from build123d import *

# Parameters (mm, degrees)
CUT_EXTRUDE_1_DEPTH      = 135.169668703
CUT_EXTRUDE_1_DEPTH_BACK = 135.169668703
SKETCH_4_R               = 3
SKETCH_5_R               = 1.5
CUT_EXTRUDE_2_DEPTH      = 10
CHAMFER_1_SIZE           = 1


with BuildPart() as part:
    # 草图1 → 旋转1 (revolve)
    with BuildSketch(Plane.XY, mode=Mode.PRIVATE) as revolve_1_sk:
        Polygon((0, 0), (0, 8), (-73.934886909, 8), (-73.934886909, 7.5), (-75.934886909, 7.5), (-75.934886909, 12.5), (-84.5, 12.5), (-84.5, 8.5), (-86.5, 8.5), (-86.5, 9), (-118, 9), (-118, 7), (-120.5, 7), (-120.5, 8), (-133, 8), (-133, 0), align=None)
    revolve(revolve_1_sk.sketch.rotate(Axis((0, 0, 0), (1, 0, 0)), 90), axis=Axis((0, 0, 0), (1, 0, 0)))

    # 草图3 → 切除-旋转3 (revolve, cut)
    with BuildSketch(Plane.XY, mode=Mode.PRIVATE) as cut_revolve_3_sk:
        with BuildLine():
            Line((-133, 3.866025404), (-131.5, 3))
            Line((-131.5, 3), (-125, 3))
            Line((-125, 3), (-125, 1.5))
            Line((-125, 1.5), (-75, 1.5))
            ThreePointArc((-75, 1.5), (-73.939339828, 1.060660172), (-73.5, 0))
            Line((-73.5, 0), (-133, 0))
            Line((-133, 0), (-133, 3.866025404))
        make_face()
    revolve(cut_revolve_3_sk.sketch.rotate(Axis((-133, 0, 0), (1, 0, 0)), 90), axis=Axis((-133, 0, 0), (1, 0, 0)), mode=Mode.SUBTRACT)

    # 草图4 → 切除-拉伸1 (cut, two sides: drawn at the far end of the back side and taken through both)
    with BuildSketch(Plane.XY.offset(-CUT_EXTRUDE_1_DEPTH_BACK)):
        with Locations((-11.434886909, 0)):
            Circle(SKETCH_4_R)
    extrude(amount=CUT_EXTRUDE_1_DEPTH + CUT_EXTRUDE_1_DEPTH_BACK, mode=Mode.SUBTRACT)

    # 草图5 → 切除-拉伸2 (cut)
    with BuildSketch(Plane.XY):
        with Locations((-75, 0)):
            Circle(SKETCH_5_R)
    extrude(amount=CUT_EXTRUDE_2_DEPTH, mode=Mode.SUBTRACT)

    # 倒角1
    chamfer_1_edges = [part.edges().sort_by_distance(p)[0] for p in [
        (-133, 0, -8),
    ]]
    chamfer(chamfer_1_edges, length=CHAMFER_1_SIZE)


solid = part.part
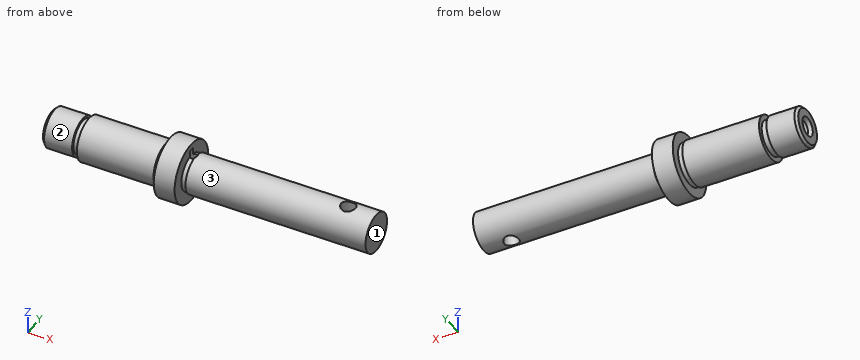
Input: part model. Units: mm. Frame: model coordinates. Face numbers are marked on the shaded views. A direction names the side the tool comes from. Coordinates: 2 decimals unless noted, no trailing zeros. Loops run counter-clockwise (first coordinate to the right, second up) from the corner with the lowest first, then second, coordinate; pieces in that order, holes last. Notation, with made-up numbers: (-27, 31.5) -> (24, 31.5) arc R31 cw to (24, 63.5) -> close; hole circle Ø11 at (66.25, 46.25). An arc over 180 degrees is marked (long way). One line per item, written item: value.
(1) Cut plane A-A (x = -34). Output: boundary loops of the cut face in (y, z), then the cut area to 3 significant figures.
Answer below:
outline: circle Ø16 at (0, 0)
area: 201 mm2
(2) Pin query (flat end, axial travel): pin 1 Ø7.5 at (y, z) = (1, -1) entering from +X; pin 2 Ø4 at (y, z) = (0, 0) entering from -X; pin 3 Ø1 at (x, y) = (-49.5, -4.5) entering from +Z; pin 4 Ø5 at (x, z) = (-35.5, -2) entering from -Y. Return the tip coordinate at first contact, or that it passes through.
Answer below:
pin 1: stops at x = 0
pin 2: stops at x = -125
pin 3: stops at z = 6.93
pin 4: stops at y = -8
(3) Set-up query: the marked faces 1, 2 and 3. Return all of +Z, -Z, +X, -X, +Y, -Y with unobstructed straight access to the full face (end or side cutting, diameter ignored); none if empty.
Answer below:
face 1: +Z, -Z, +X, +Y, -Y
face 2: -X
face 3: +X
(4) Ray query, line 1 along Y through (x, z) = (-126.25, 0); line 2 along X through (y, z) = (0, -5); line 3 along Y through (x, z) = (-99, 0). Return the intervals inside material, ascending.
Answer below:
line 1: y = -8 to -3, 3 to 8
line 2: x = -133 to -14.43, -8.43 to 0
line 3: y = -9 to -1.5, 1.5 to 9
